Read the model definition and answer for the solid it produces. Units are mm, in the model's axes. A direction names the side the tool comes from. Give positions to 0.01 mm unless a question says otherwise; leave off trailing zeros. Loops run counter-clockwise (first coordinate to the right, second up) from the corner with the lowest first, then second, coordinate; pieces in that order, holes last.
(1) Find section D-D, the plane y = 391. Write down the section's boundary in (x, z) (3 decimals).
(2) Find section A-A, the plane y = 460. Write down the section's boundary in (x, z) (3 decimals), then the cut area to 3 significant figures.
(3) Find section C-C, the plane z = -53.5. Write down the section's boundary in (x, y) (3 decimals), then the cut area to 3 significant figures.
(4) Each of these flat-tipped pins is pushed along its axis until it touches: P1, Ø1, axis at x = 313.5, y = 232.5, coming from the -Z side (3 decimals); P2, Ø12, axis at y = 258, z = 33.5, coming from the -X side; P3, Ø12, axis at x = 100.5, y = 395.5, coming from the -Z side. Where does it stop, or does it pass through?
(5) Straight lines are drawn through the part: probe 1 along Z at (x, y) = (69, 276.5) (3 decimals); probe 2 along Y at (x, z) = (117, -31.5) (3 decimals); probe 3 along Z at (x, y) = (-239, 311) (3 decimals). For each, find the intervals that lie inside material, in ascending order.
(6) Which of the six approach directions +Z, -Z, +X, -X, +Y, -Y give full straight-line access (tool end or side, diameter ignored) to faces 5 (the face through (-2, 200, 127)), 6 (the face through (252.578, 200.355, 64.389)), 7 (the face through (2, 204, -123.825)), 8 (the face through (2, 200, -127)), 9 (the face through (-255.422, 200.355, 62.611))?
(7) Find section B-B, the plane x = -139.5. Write down the section's boundary in (y, z) (3 decimals), then the cut area to 3 significant figures.
(8) Determine the mould class of faces 1 (the face through (255.422, 200.355, -62.611)), 2 (the face through (-273.068, 459.664, -74.047)), 3 (the face through (-5, 0, -2)), 4 (the face through (276.48, 458.05, 75.66)) for opening direction Z: pulls with the +Z half, pulls with the -Z half, needs draft (parallel to the pull), parting line crosses it, or undercut.
```python
from build123d import *

# Parameters (mm, degrees)
BOSS_EXTRUDE1_DEPTH = 3.175
BOSS_EXTRUDE2_DEPTH = 403.225
BOSS_EXTRUDE3_DEPTH = 3.175
BOSS_EXTRUDE4_DEPTH = 101.6


with BuildPart() as part:
    # Sketch2 → Boss-Extrude1 (new body)
    with BuildSketch(Plane(origin=(0, 0, 0), x_dir=(1, 0, 0), z_dir=(0, 1, 0))):
        Polygon((-152.4, 127), (-355.6, 0), (-152.4, -127), (152.4, -127), (355.6, 0), (152.4, 127), align=None)
    extrude(amount=BOSS_EXTRUDE1_DEPTH)

    # Sketch3 → Boss-Extrude2 (add)
    with BuildSketch(Plane(origin=(0, 3.175, 0), x_dir=(1, 0, 0), z_dir=(0, 1, 0))):
        Polygon((152.4, -127), (355.6, 0), (152.4, 127), (-152.4, 127), (-355.6, 0), (-152.4, -127), align=None)
        Polygon((151.489421981, -123.825), (349.609421981, 0), (151.489421981, 123.825), (-151.489421981, 123.825), (-349.609421981, 0), (-151.489421981, -123.825), align=None, mode=Mode.SUBTRACT)
    extrude(amount=BOSS_EXTRUDE2_DEPTH)

    # Sketch5 → Boss-Extrude3 (add)
    with BuildSketch(Plane(origin=(0, 406.4, 0), x_dir=(1, 0, 0), z_dir=(0, 1, 0))):
        Polygon((158.774046132, 149.225), (-158.774046132, 149.225), (-397.534046132, 0), (-158.774046132, -149.225), (158.774046132, -149.225), (397.534046132, 0), align=None)
        Polygon((151.489421981, 123.825), (-151.489421981, 123.825), (-349.609421981, 0), (-151.489421981, -123.825), (151.489421981, -123.825), (349.609421981, 0), align=None, mode=Mode.SUBTRACT)
    extrude(amount=BOSS_EXTRUDE3_DEPTH)

    # Sketch6 → Boss-Extrude4 (add)
    with BuildSketch(Plane(origin=(0, 409.575, 0), x_dir=(1, 0, 0), z_dir=(0, 1, 0))):
        Polygon((-158.774046132, 149.225), (-397.534046132, 0), (-158.774046132, -149.225), (158.774046132, -149.225), (397.534046132, 0), (158.774046132, 149.225), align=None)
        Polygon((-157.863468113, 146.05), (-391.543468113, 0), (-157.863468113, -146.05), (157.863468113, -146.05), (391.543468113, 0), (157.863468113, 146.05), align=None, mode=Mode.SUBTRACT)
    extrude(amount=BOSS_EXTRUDE4_DEPTH)


solid = part.part
```
Entries:
1. outline: (-355.6, 0) - (-152.4, -127) - (152.4, -127) - (355.6, 0) - (152.4, 127) - (-152.4, 127) - close; hole (-349.609, 0) - (-151.489, -123.825) - (151.489, -123.825) - (349.609, 0) - (151.489, 123.825) - (-151.489, 123.825) - close
2. outline: (-397.534, 0) - (-158.774, -149.225) - (158.774, -149.225) - (397.534, 0) - (158.774, 149.225) - (-158.774, 149.225) - close; hole (-391.543, 0) - (-157.863, -146.05) - (157.863, -146.05) - (391.543, 0) - (157.863, 146.05) - (-157.863, 146.05) - close
2. area: 5,550 mm2
3. outline: (-311.934, 406.4) - (-270, 406.4) - (-270, 0) - (270, 0) - (270, 406.4) - (311.934, 406.4) - (311.934, 511.175) - (305.943, 511.175) - (305.943, 409.575) - (264.009, 409.575) - (264.009, 3.175) - (-264.009, 3.175) - (-264.009, 409.575) - (-305.943, 409.575) - (-305.943, 511.175) - (-311.934, 511.175) - close
3. area: 8,070 mm2
4. P1: stops at z = -26.625
4. P2: stops at x = -311.6
4. P3: stops at z = -127
5. probe 1: z = -127 to -123.825, 123.825 to 127
5. probe 2: y = 0 to 3.175
5. probe 3: z = -72.875 to -69.131, 69.131 to 72.875
6. face 5: +Z, +X, -X, -Y
6. face 6: +Z, +X, -Y
6. face 7: +Y
6. face 8: -Z, +X, -X, -Y
6. face 9: +Z, -X, -Y
7. outline: (0, -127) - (406.4, -127) - (406.4, -149.225) - (511.175, -149.225) - (511.175, -146.05) - (409.575, -146.05) - (409.575, -123.825) - (3.175, -123.825) - (3.175, 123.825) - (409.575, 123.825) - (409.575, 146.05) - (511.175, 146.05) - (511.175, 149.225) - (406.4, 149.225) - (406.4, 127) - (0, 127) - close
7. area: 4,170 mm2
8. face 1: pulls with the -Z half
8. face 2: undercut
8. face 3: needs draft
8. face 4: pulls with the +Z half
